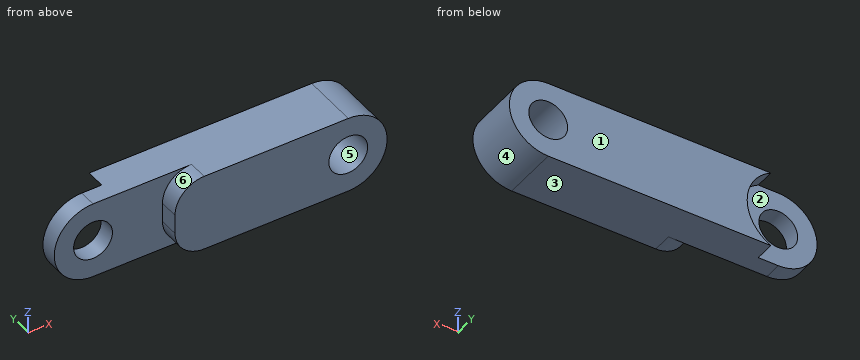
```python
from build123d import *

# Parameters (mm, degrees)
SKETCH1_R           = 20
BOSS_EXTRUDE1_DEPTH = 58
SKETCH3_R           = 45
CUT_EXTRUDE2_DEPTH  = 20
CUT_EXTRUDE3_START  = -20
SKETCH4_R           = 45
CUT_EXTRUDE3_DEPTH  = 20
SKETCH6_W           = 142.996364582
SKETCH6_H           = 80
CUT_EXTRUDE6_DEPTH  = 20
FILLET1_R           = 30


with BuildPart() as part:
    # Sketch1 → Boss-Extrude1 (new body)
    with BuildSketch(Plane(origin=(0, 0, 0), x_dir=(1, 0, 0), z_dir=(0, 1, 0))):
        with BuildLine():
            Line((-125, 40), (125.000000012, 40))
            ThreePointArc((125.000000012, 40), (165, -6e-09), (125, -40))
            Line((125, -40), (-125, -40))
            ThreePointArc((-125, -40), (-165, 0), (-125, 40))
        make_face()
        with Locations(Location((-125, 0, 0), (0, 0, 90))):
            Circle(SKETCH1_R, mode=Mode.SUBTRACT)
        with Locations(Location((125, 0, 0), (0, 0, 90))):
            Circle(SKETCH1_R, mode=Mode.SUBTRACT)
    extrude(amount=BOSS_EXTRUDE1_DEPTH)

    # Sketch3 → Cut-Extrude2 (cut)
    with BuildSketch(Plane(origin=(0, 58, 0), x_dir=(1, 0, 0), z_dir=(0, 1, 0))):
        with Locations((-125, 0)):
            Circle(SKETCH3_R)
    extrude(amount=-CUT_EXTRUDE2_DEPTH, mode=Mode.SUBTRACT)

    # Sketch4 → Cut-Extrude3 (cut)
    with BuildSketch(Plane.XZ.offset(CUT_EXTRUDE3_START)):
        with Locations((-125, 0)):
            Circle(SKETCH4_R)
    extrude(amount=CUT_EXTRUDE3_DEPTH, mode=Mode.SUBTRACT)

    # Sketch6 → Cut-Extrude6 (cut)
    with BuildSketch(Plane.XZ):
        with Locations((-125, 0)):
            Rectangle(SKETCH6_W, SKETCH6_H)
    extrude(amount=-CUT_EXTRUDE6_DEPTH, mode=Mode.SUBTRACT)

    # Fillet1
    fillet1_edges = [part.edges().sort_by_distance(p)[0] for p in [
        (-53.501817709, 10, -40),
        (-53.501817709, 10, 40),
    ]]
    fillet(fillet1_edges, radius=FILLET1_R)


solid = part.part
```
CAD build for the part. Positions are in the model's coordinates, mm. Face numbers are marked on the shaded views. A direction names the side the tool comes from. Coordinates: 2 decimals unless noted, no trailing zeros. Order: outer loops, then holes, each group sorted by start corner. A loop starts at its lowest first (then second) coordinate and runs counter-clockwise, first axis right, second up. Notation, with made-up numbers: (-14, 9) -> (-8, 9) arc R17 ccw to (-8, 21) -> close; hole circle Ø1 at (-20.5, -4). An arc over 180 degrees is marked (long way). Use one line per item in the form item = value. Start each with the question number.
1) Band-saw the part on C-C on x = -115. Give the cut face in (y, z).
2) Pull direction X, two halves, no side cores. Call the marked faces 3, 4, 5 and 6: +X half, -X half, draft (parallel to the pull), parting line (faces both ways), or undercut.
3) Drop flat-ended pins along their axis: pin 1 (24 mm diameter, centred on x = -125, z = 0, fed in from -Y); pin 2 (3 mm diameter, centred on x = -58.5, z = 31.5, fed in from -Y); pin 3 (3 mm diameter, centred on y = 16.5, z = 7, fed in from -X). Give the stop position or say it passes through.
4) Band-saw the part on B-B on y = 28.5. Give the cut face in (x, z).
5) Band-saw the part on D-D on y = 9.5. Give the cut face in (x, z).
6) Drill centre lines: L1, parallel to X at y = 33.5, z = 0; L2, parallel to X at y = 22, z = 3.5; L3, parallel to X at y = 39.5, z = 0. Where is each one in solid material? Low to high. Write a range as [from, to].
7) Band-saw the part on A-A on z = 0. Give the cut face in (x, y), then the cut area to 3 significant figures.
8) Tool access for the marked faces 1 and 2: list every direction of +Z, -Z, +X, -X, +Y, -Y with a clear straight run to the whole face (end or side of a thin tool).
Entries:
q1.outline = (20, -40) -> (38, -40) -> (38, -17.32) -> (20, -17.32) -> close; (20, 17.32) -> (38, 17.32) -> (38, 40) -> (20, 40) -> close
q2.face_3 = draft
q2.face_4 = +X half
q2.face_5 = undercut
q2.face_6 = -X half
q3.pin_1 = through
q3.pin_2 = 20
q3.pin_3 = -53.5
q4.outline = (-125, -40) -> (125, -40) arc R40 ccw to (125, 40) -> (-125, 40) arc R40 ccw to start; hole circle Ø40 at (-125, 0); hole circle Ø40 at (125, 0)
q5.outline = (-53.5, -10) arc R30 ccw to (-23.5, -40) -> (125, -40) arc R40 ccw to (125, 40) -> (-23.5, 40) arc R30 ccw to (-53.5, 10) -> close; hole circle Ø40 at (125, 0)
q6.L1 = [-165, -145], [-105, 105], [145, 165]
q6.L2 = [-164.85, -144.69], [-105.31, 105.31], [144.69, 164.85]
q6.L3 = [-80, 105], [145, 165]
q7.outline = (-165, 20) -> (-145, 20) -> (-145, 38) -> (-165, 38) -> close; (-105, 20) -> (-53.5, 20) -> (-53.5, 0) -> (105, 0) -> (105, 58) -> (-80, 58) -> (-80, 38) -> (-105, 38) -> close; (145, 0) -> (165, 0) -> (165, 58) -> (145, 58) -> close
q7.area = 12,200 mm2
q8.face_1 = +Z, -Z, +X, -X, +Y
q8.face_2 = -X, +Y
